Geometry check sheet. Reference: the model listing, model coordinates, mm. Face numbers are marked on the shaded views. Coordinates: 2 decimals unless noted, no trailing zeros. Order: outer loops, then holes, each group sorted by start corner. A loop starts at its lowest first (then second) coordinate and runs counter-clockwise, first axis right, second up. Notation, with made-up numbers: (9.5, -36) - (28.5, -36) arc R24 ccw to (28.5, -21) - close; hole circle Ø2 at (54.5, 21.25). An arc over 180 degrees is marked (long way). Use CSV: the item, a comma, the result in double quotes. Start each with the question number.
1) Draft check along Z on the marked faces 1, 2 and 3. Enter one of: released by +Z, released by -Z, zero draft, split by the parting line, or undercut.
2) Sectioned sample at A-A, the plane y = 0. Record the cut outline in (x, z), and give its area (3 significant figures).
3) Thickness scan on probe 1 along Z at (x, y) = (2, 7); probe 2 along Z at (x, y) = (2.5, -5); probe 3 along Z at (x, y) = (2.75, 8.5). Record the ranges inside material, lowest first. Write a range as [from, to].
4) Sectioned sample at B-B, the plane z = -26. Record the cut outline in (x, y) (3 decimals), and give its area (3 significant figures).
5) Sectioned sample at C-C, the plane x = 3.25. Count the separate pieces of the cut face and the enclosed holes in it, and give its area (3 significant figures).
6) Depth check by flat-ended pin: P1, Ø3, axis at x = 5, z = -34, coming from the +Y side (3 decimals); P2, Ø4, axis at y = 0, z = -20.066, coming from the +X side; P3, Ø4, axis at x = 2.5, z = -24, coming from the -Y side (3 decimals); P4, Ø3.5, axis at x = 5.5, y = -20.5, coming from the -Z side. Enter the tip coordinate at first touch or a pass-through.
7) Sectioned sample at D-D, the plane z = -40.5. Record the cut outline in (x, y) (3 decimals), and give its area (3 significant figures).
from build123d import *

# Parameters (mm, degrees)
SKETCH1_W           = 45.7835
SKETCH1_H           = 21.082
SKETCH1_R           = 1.905
BOSS_EXTRUDE1_DEPTH = 5.08
SKETCH2_R           = 1.905
BOSS_EXTRUDE2_DEPTH = 3.175
SKETCH4_W           = 31.75
SKETCH4_H           = 38.1
SKETCH4_R           = 6.4008
SKETCH4_R_2         = 2.286
BOSS_EXTRUDE4_DEPTH = 5.08


with BuildPart() as part:
    # Sketch1 → Boss-Extrude1 (new body)
    with BuildSketch(Plane.YZ):
        Rectangle(SKETCH1_W, SKETCH1_H)
        with Locations(Location((-20.28825, -7.9375, 0), (0, 0, 270))):
            Circle(SKETCH1_R, mode=Mode.SUBTRACT)
        with Locations(Location((20.28825, 7.9375, 0), (0, 0, 270))):
            Circle(SKETCH1_R, mode=Mode.SUBTRACT)
    extrude(amount=BOSS_EXTRUDE1_DEPTH)

    # Sketch2 → Boss-Extrude2 (add)
    # profile 1 of 2: a face of its own
    with BuildSketch(Plane.YZ.offset(5.08)):
        with BuildLine():
            Line((18.470995821, 10.541), (22.105504179, 10.541))
            ThreePointArc((22.105504179, 10.541), (22.53331403, 10.18256403), (22.89175, 9.754754179))
            Line((22.89175, 9.754754179), (22.89175, 6.120245821))
            ThreePointArc((22.89175, 6.120245821), (18.04318597, 5.69243597), (18.470995821, 10.541))
        make_face()
        with Locations(Location((20.28825, 7.9375, 0), (0, 0, 270))):
            Circle(SKETCH2_R, mode=Mode.SUBTRACT)
    # profile 2 of 2: a face of its own
    with BuildSketch(Plane.YZ.offset(5.08)):
        with BuildLine():
            Line((-22.89175, -6.120245821), (-22.89175, -9.754754179))
            ThreePointArc((-22.89175, -9.754754179), (-22.53331403, -10.18256403), (-22.105504179, -10.541))
            Line((-22.105504179, -10.541), (-18.470995821, -10.541))
            ThreePointArc((-18.470995821, -10.541), (-18.04318597, -5.69243597), (-22.89175, -6.120245821))
        make_face()
        with Locations(Location((-20.28825, -7.9375, 0), (0, 0, 270))):
            Circle(SKETCH2_R, mode=Mode.SUBTRACT)
    extrude(amount=BOSS_EXTRUDE2_DEPTH)

    # Sketch4 → Boss-Extrude4 (add)
    with BuildSketch(Plane(origin=(0, 0, 0), x_dir=(0, -1, 0), z_dir=(-1, 0, 0))):
        with Locations((0, -29.591)):
            Rectangle(SKETCH4_W, SKETCH4_H)
        with Locations(Location((0, -29.591, 0), (0, 0, 90))):
            Circle(SKETCH4_R, mode=Mode.SUBTRACT)
        with Locations(Location((0, -20.066, 0), (0, 0, 90))):
            Circle(SKETCH4_R_2, mode=Mode.SUBTRACT)
        with Locations(Location((6.735192091, -22.855807909, 0), (0, 0, 90))):
            Circle(SKETCH4_R_2, mode=Mode.SUBTRACT)
        with Locations(Location((9.525, -29.591, 0), (0, 0, 90))):
            Circle(SKETCH4_R_2, mode=Mode.SUBTRACT)
        with Locations(Location((6.735192091, -36.326192091, 0), (0, 0, 90))):
            Circle(SKETCH4_R_2, mode=Mode.SUBTRACT)
        with Locations(Location((0, -39.116, 0), (0, 0, 90))):
            Circle(SKETCH4_R_2, mode=Mode.SUBTRACT)
        with Locations(Location((-6.735192091, -36.326192091, 0), (0, 0, 90))):
            Circle(SKETCH4_R_2, mode=Mode.SUBTRACT)
        with Locations(Location((-9.525, -29.591, 0), (0, 0, 90))):
            Circle(SKETCH4_R_2, mode=Mode.SUBTRACT)
        with Locations(Location((-6.735192091, -22.855807909, 0), (0, 0, 90))):
            Circle(SKETCH4_R_2, mode=Mode.SUBTRACT)
    extrude(amount=-BOSS_EXTRUDE4_DEPTH)


solid = part.part
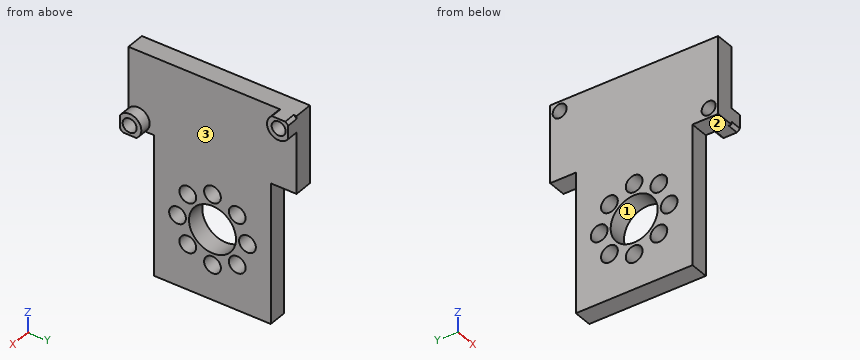
Evaluation:
1,face 1,"undercut"
1,face 2,"released by -Z"
1,face 3,"zero draft"
2,outline,"(0, -48.64) - (5.08, -48.64) - (5.08, -41.4) - (0, -41.4) - close; (0, -36.83) - (5.08, -36.83) - (5.08, -35.99) - (0, -35.99) - close; (0, -23.19) - (5.08, -23.19) - (5.08, -22.35) - (0, -22.35) - close; (0, -17.78) - (5.08, -17.78) - (5.08, 10.54) - (0, 10.54) - close"
2,area,"189 mm²"
3,probe 1,"[-48.64, -38.6], [-34.06, -25.13], [-20.59, 10.54]"
3,probe 2,"[-48.64, -37.81], [-34.84, -33.59], [-25.59, -24.34], [-21.37, 10.54]"
3,probe 3,"[-48.64, -37.78], [-34.87, -31.63], [-27.55, -24.31], [-21.4, 10.54]"
4,outline,"(0, -15.875) - (5.08, -15.875) - (5.08, -5.299) - (0, -5.299) - close; (0, 5.299) - (5.08, 5.299) - (5.08, 15.875) - (0, 15.875) - close"
4,area,"107 mm²"
5,separate pieces,"1"
5,enclosed holes,"11"
5,area,"1,890 mm²"
6,P1,"y = 15.875"
6,P2,"through"
6,P3,"y = -15.875"
6,P4,"z = -10.54"
7,outline,"(0, -15.875) - (5.08, -15.875) - (5.08, -1.819) - (0, -1.819) - close; (0, 1.819) - (5.08, 1.819) - (5.08, 15.875) - (0, 15.875) - close"
7,area,"143 mm²"
